from build123d import *

# Parameters (mm, degrees)
SKETCH_1_W          = 76
SKETCH_1_H          = 53
SKETCH_1_R          = 1.55
EXTRUDE_1_DEPTH     = 1.5
SKETCH_2_W          = 76
SKETCH_2_H          = 1.5
EXTRUDE_2_DEPTH     = 1.5
SKETCH_3_W          = 76
SKETCH_3_H          = 1.5
EXTRUDE_3_DEPTH     = 35.02
SKETCH_4_R          = 5.36
SKETCH_4_R_2        = 2.600000007
CUT_EXTRUDE_1_DEPTH = 60


with BuildPart() as part:
    # 草图1 → 凸台-拉伸1 (new body)
    with BuildSketch(Plane(origin=(0, 0, 0), x_dir=(1, 0, 0), z_dir=(0, 1, 0))):
        Rectangle(SKETCH_1_W, SKETCH_1_H)
        with Locations((-34.29, 22.86)):
            Circle(SKETCH_1_R, mode=Mode.SUBTRACT)
        with Locations((-34.29, -22.86)):
            Circle(SKETCH_1_R, mode=Mode.SUBTRACT)
        with Locations((34.29, -22.86)):
            Circle(SKETCH_1_R, mode=Mode.SUBTRACT)
        with Locations((34.29, 22.86)):
            Circle(SKETCH_1_R, mode=Mode.SUBTRACT)
    extrude(amount=EXTRUDE_1_DEPTH)

    # 草图2 → 凸台-拉伸2 (add)
    with BuildSketch(Plane.XY.offset(26.5)):
        with Locations((0, 0.75)):
            Rectangle(SKETCH_2_W, SKETCH_2_H)
    extrude(amount=EXTRUDE_2_DEPTH)

    # 草图3 → 凸台-拉伸3 (add)
    with BuildSketch(Plane(origin=(0, 1.5, 0), x_dir=(1, 0, 0), z_dir=(0, 1, 0))):
        with Locations((0, -27.25)):
            Rectangle(SKETCH_3_W, SKETCH_3_H)
    extrude(amount=EXTRUDE_3_DEPTH)

    # 草图4 → 切除-拉伸1 (cut)
    with BuildSketch(Plane(origin=(0, 0, 26.5), x_dir=(-1, 0, 0), z_dir=(0, 0, -1))):
        with Locations((0, 19.02)):
            Circle(SKETCH_4_R)
        with Locations((-12.7, 19.02)):
            Circle(SKETCH_4_R_2)
        with Locations((-25.4, 19.02)):
            Circle(SKETCH_4_R_2)
        with Locations((12.7, 19.02)):
            Circle(SKETCH_4_R_2)
        with Locations((25.4, 19.02)):
            Circle(SKETCH_4_R_2)
    extrude(amount=-CUT_EXTRUDE_1_DEPTH, mode=Mode.SUBTRACT)


solid = part.part
Work out the finished part from the listing and answer in its coordinate system (mm). A direction names the side the tool comes from. Round coordinates to 2 decimals unless told otherwise and drop trailing zeros. Order: outer loops, then holes, each group sorted by start corner. A loop starts at its lowest first (then second) coordinate and runs counter-clockwise, first axis right, second up. Notation, with made-up numbers: M 75.5,-26 L 130.5,-26 A22 cw 130.5,-5 Z; hole C -40,14.25 d4. An arc over 180 degrees is marked long. Put each result on its own line as item: value. Start each with the question number.
Q1. Section D-D, the plane z = -19 is taken. Write down the section's boundary in (x, y), and give its area (3 significant figures).
Q2. Section A-A, the plane x = 12.7 is taken. Write down the section's boundary in (y, z), and give its area (3 significant figures).
Q3. Section C-C, the plane x = -34.29 is taken. Write down the section's boundary in (y, z).
Q4. Flat-ended cylindrical pins translate along their axes: pin 1 (4 mm diameter, centred on x = -25.4, y = 19.02, fed in from -Z); pin 2 (10 mm diameter, centred on x = 19.5, y = 26.5, fed in from -Z); pin 3 (4 mm diameter, centred on x = 34.29, z = -22.86, fed in from +Y). Find the tip coordinate at first contact, or state that the pin passes through.
Q5. Section B-B, the plane z = 22.86 is taken. Write down the section's boundary in (x, y).
Q6. Straight lines are drawn through the part: L1, parallel to Z at x = 34.29, y = 0.7; L2, parallel to X at y = 19, z = 27; L3, parallel to Y at x = 0, z = 27.5. For each, find the intervals that lie inside material, in ascending order. Write a range as [from, to].
Q7. For a pull along Z with two mould halves and no side action, classify faces 1 (the cylindrical face through (0.698, 24.334, 27.24)), 2 (the flat face through (-1, 26, 28)), 3 (the cylindrical face through (35.005, 0.74, -21.485)) as pulls with the +Z half, pulls with the -Z half, needs draft (parallel to the pull), parting line crosses it, or undercut.
Q8. A tool of negligible diameter and unlimited length cuts with its end or side. For faces 4 (the cylindrical face through (24.2, 16.713, 27.24)), 5 (the flat face through (-1, 11, 26.5)), from which of +Z, -Z, +X, -X, +Y, -Y can it reach the whole face along a straight path? Write none if from no direction.
Findings below:
1. outline: M -38,0 L 38,0 L 38,1.5 L -38,1.5 Z
1. area: 114 mm^2
2. outline: M 0,-26.5 L 1.5,-26.5 L 1.5,26.5 L 16.42,26.5 L 16.42,28 L 0,28 Z; M 21.62,26.5 L 36.52,26.5 L 36.52,28 L 21.62,28 Z
2. area: 126 mm^2
3. outline: M 0,-26.5 L 1.5,-26.5 L 1.5,-24.41 L 0,-24.41 Z; M 0,-21.31 L 1.5,-21.31 L 1.5,21.31 L 0,21.31 Z; M 0,24.41 L 1.5,24.41 L 1.5,26.5 L 36.52,26.5 L 36.52,28 L 0,28 Z
4. pin 1: passes through
4. pin 2: stops at z = 26.5
4. pin 3: stops at y = 1.5
5. outline: M -38,0 L -35.84,0 L -35.84,1.5 L -38,1.5 Z; M -32.74,0 L 32.74,0 L 32.74,1.5 L -32.74,1.5 Z; M 35.84,0 L 38,0 L 38,1.5 L 35.84,1.5 Z
6. L1: z = [-26.5, -24.41], [-21.31, 21.31], [24.41, 28]
6. L2: x = [-38, -28], [-22.8, -15.3], [-10.1, -5.36], [5.36, 10.1], [15.3, 22.8], [28, 38]
6. L3: y = [0, 13.66], [24.38, 36.52]
7. face 1: needs draft
7. face 2: pulls with the +Z half
7. face 3: undercut
8. face 4: +Z, -Z
8. face 5: -Z, +X, -X, +Y
